Can you work these out from the model? Positions are in its coordinate system, mm. A direction names the side the tool comes from. Coordinates: 2 decimals unless noted, no trailing zeros. Order: outer loops, then holes, each group sorted by start corner. A loop starts at its lowest first (then second) coordinate and runs counter-clockwise, first axis right, second up. Notation, with made-up numbers: (-1.75, 38.25) -> (7.25, 38.25) arc R19 cw to (7.25, 62.25) -> close; hole circle Ø3 at (27, -32). An arc over 180 degrees is marked (long way). Answer as a JSON object with one key per item and string values. Group by question number.
(1) Which directions (+Z, -Z, +X, -X, +Y, -Y) give clear straight access to the entire face, cutting with the end or side of a thin tool? Please do faces 1 (the flat face through (-3.8, 8.4, 0)), 2 (the flat face through (8, -5, 22)).
(2) For pin 1 (5 mm diameter, centred on x = 10, z = 20.5, fed in from +Y); pin 2 (1.4 mm diameter, centred on x = -7.5, y = 5.5, fed in from -Z); pin 3 (5 mm diameter, centred on y = 3.5, z = 13.5, fed in from -X); pin 4 (2 mm diameter, centred on x = 1.5, y = -6.5, fed in from +Z), each with a flat end and sliding along its axis, tell me the tip position at first contact or that it passes through.
(3) I want a section at A-A, the plane z = 12.5. List the corners of the cut face in (x, y) for me, plus the area to 3 significant figures.
(4) If we mould it in two halves opening along Y, with no side actions, what happens to faces 3 (the flat face through (4.44, 7.83, 10.85)), 4 (the cylindrical face through (11.923, 3.755, 10.846)), 5 (the flat face through (0, 0, 32))? For each: pulls with the +Y half, pulls with the -Y half, needs draft (parallel to the pull), parting line crosses it, or undercut.
(5) I need wall thicknesses on line 1 (Y direction, x = 0, z = 19); line 2 (Y direction, x = 4, z = 25); line 3 (X direction, y = -6, z = 23.5). Which ranges of each line are inside material? Lowest first, please.
from build123d import *

# Parameters (mm, degrees)
F0_R     = 12.5
F1_DEPTH = 22
F3_DEPTH = 22
F4_R     = 12.5
F5_DEPTH = 10
F6_R     = 10
F8_DEPTH = 5
F9_R     = 4.99999


# Not quite as in the source:
# - a fillet or chamfer is up to 0.001 mm smaller than in the source, because OpenCascade refuses the exact size


with BuildPart() as f1:
    # F0 (on Top) → F1 (new body)
    with BuildSketch(Plane.XY):
        Circle(F0_R)
    extrude(amount=F1_DEPTH)

    # F2 (on face) → F3 (cut, through all)
    with BuildSketch(Plane(origin=(0, 0, 0), x_dir=(1, 0, 0), z_dir=(0, 0, -1))):
        Polygon((9, -5.1961524227), (9, 5.1961524227), (0, 10.3923048454), (-9, 5.1961524227), (-9, -5.1961524227), (0, -10.3923048454), align=None)
    extrude(amount=-F3_DEPTH, mode=Mode.SUBTRACT)

    # F4 (on face) → F5 (join)
    with BuildSketch(Plane.XY.offset(22)):
        Circle(F4_R)
    extrude(amount=F5_DEPTH)

    # F6
    f6_edges = [f1.edges().sort_by_distance(p)[0] for p in [
        (-12.5, 0, 32),
    ]]
    fillet(f6_edges, radius=F6_R)

    # F7 (on face) → F8 (cut)
    with BuildSketch(Plane(origin=(0, 0, 22), x_dir=(1, 0, 0), z_dir=(0, 0, -1))):
        with BuildLine():
            ThreePointArc((4.499999942, -7.7942286675), (7.7942286173, -4.500000029), (9, 0))
            ThreePointArc((9, 0), (7.7942286173, 4.500000029), (4.499999942, 7.7942286675))
            ThreePointArc((4.499999942, 7.7942286675), (-1.087e-07, 9), (-4.5000001303, 7.7942285588))
            ThreePointArc((-4.5000001303, 7.7942285588), (-7.7942286717, 4.4999999349), (-9, 0))
            ThreePointArc((-9, 0), (-7.7942286277, -4.500000011), (-4.499999978, -7.7942286468))
            ThreePointArc((-4.499999978, -7.7942286468), (-2.08e-08, -9), (4.499999942, -7.7942286675))
        make_face()
    extrude(amount=-F8_DEPTH, mode=Mode.SUBTRACT)

    # F9 (radius 5 in the source; OpenCascade refuses exactly that, so slightly less here)
    f9_edges = [f1.edges().sort_by_distance(p)[0] for p in [
        (-4.5, 7.794229, 27),
    ]]
    fillet(f9_edges, radius=F9_R)


solid = f1.part
Computed values:
{
 "1": {"face 1": "-Z, +X, -X, +Y, -Y", "face 2": "-Z"},
 "2": {"pin 1": "stops at y = 10", "pin 2": "stops at z = 0", "pin 3": "stops at x = -12.46", "pin 4": "stops at z = 31.48"},
 "3": {"outline": "circle Ø25 at (0, 0); hole (-9, -5.2) -> (0, -10.39) -> (9, -5.2) -> (9, 5.2) -> (0, 10.39) -> (-9, 5.2) -> close", "area": "210 mm2"},
 "4": {"face 3": "undercut", "face 4": "parting line crosses it", "face 5": "needs draft"},
 "5": {"line 1": "y = -12.5 to -10.39, 10.39 to 12.5", "line 2": "y = -11.36 to -6.93, 6.93 to 11.36", "line 3": "x = -10.84 to -6.4, 6.4 to 10.84"}
}
